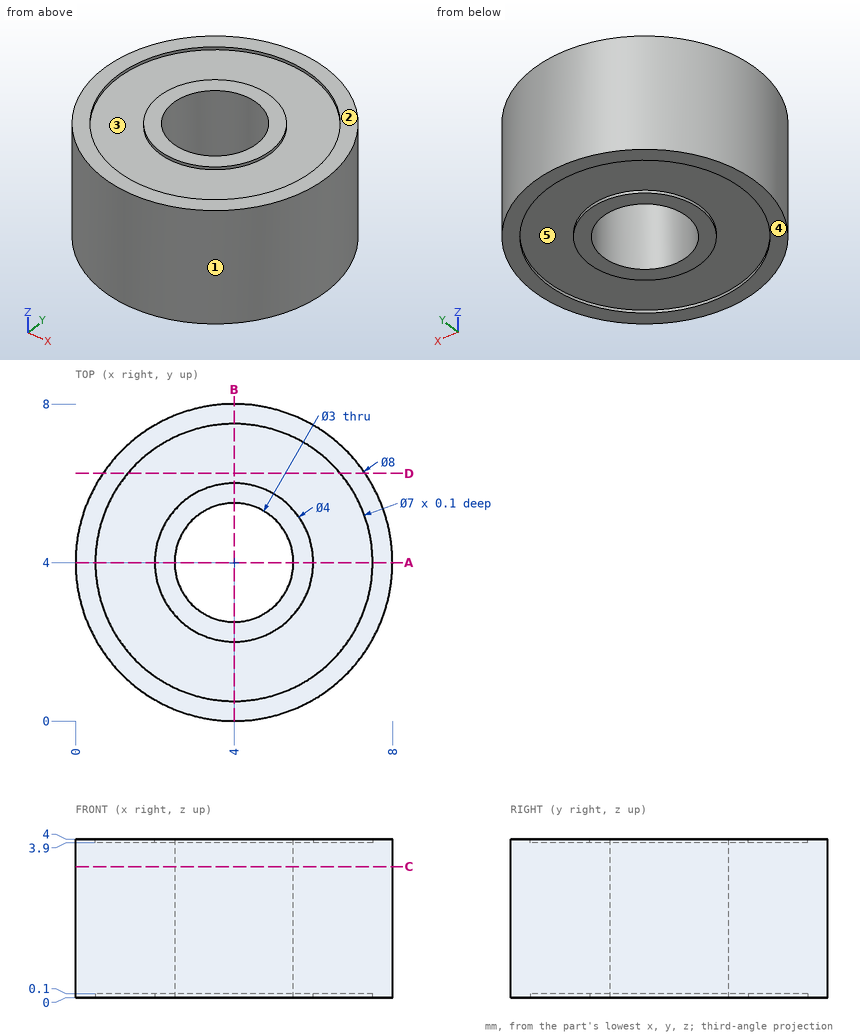
Verification items for this drawing (mm, ordinates from the low corner). A direction names the side the tool comes from. Coordinates: 2 decimals unless noted, no trailing zeros. Order: outer loops, then holes, each group sorted by start corner. A loop starts at its lowest first (then second) coordinate and runs counter-clockwise, first axis right, second up. Notation, with made-up numbers: M 38.5,30.25 L 80.5,30.25 A32 ccw 80.5,61.25 Z; hole C 21.25,79 d9. An arc over 180 degrees is marked long. Answer as a JSON object with one key per item and string values.
Q1. Cross-section at D-D on y = 6.25. Record the cut outline in (x, z).
Results are:
{"outline": "M 0.69,0 L 1.32,0 L 1.32,0.1 L 6.68,0.1 L 6.68,0 L 7.31,0 L 7.31,4 L 6.68,4 L 6.68,3.9 L 1.32,3.9 L 1.32,4 L 0.69,4 Z"}
Q2. Release check for a two-part mould opening along Y. For the marked faces 1, 2 and 3 record: released by +Y, released by -Y, zero draft, split by the parting line, or undercut.
Results are:
{"face 1": "split by the parting line", "face 2": "zero draft", "face 3": "undercut"}
Q3. Cross-section at A-A on y = 4. Record the cut outline in (x, z), and give its area (3 significant figures).
Results are:
{"outline": "M 0,0 L 0.5,0 L 0.5,0.1 L 2,0.1 L 2,0 L 2.5,0 L 2.5,4 L 2,4 L 2,3.9 L 0.5,3.9 L 0.5,4 L 0,4 Z; M 5.5,0 L 6,0 L 6,0.1 L 7.5,0.1 L 7.5,0 L 8,0 L 8,4 L 7.5,4 L 7.5,3.9 L 6,3.9 L 6,4 L 5.5,4 Z", "area": "19.4 mm²"}
Q4. Cross-section at C-C on z = 3.3. Record the cut outline in (x, y).
Results are:
{"outline": "C 4,4 d8; hole C 4,4 d3"}
Q5. Tool access check on the marked faces 4 and 5. Record the directions out of +Z, -Z, +X, -X, +Y, -Y that give a thin tool (end or side, any length) a straight path to the whole face; none if there is none.
Results are:
{"face 4": "-Z, +X, -X, +Y, -Y", "face 5": "-Z"}
Q6. Scan lines: line 1 (Y direction, x = 4, z = 0.05); line 2 (Y direction, x = 4, z = 2.25); line 3 (Z direction, x = 5, y = 6.75). Record each from-to range of solid material in increasing order.
Results are:
{"line 1": "y = 0 to 0.5, 2 to 2.5, 5.5 to 6, 7.5 to 8", "line 2": "y = 0 to 2.5, 5.5 to 8", "line 3": "z = 0.1 to 3.9"}
Q7. Depth check by flat-ended pin: pin 1 Ø2 at (x, y) = (2.5, 5) entering from -Z; pin 2 Ø2 at (y, z) = (5.5, 3) entering from -X; pin 3 Ø1 at (y, z) = (2, 1.5) entering from +X. Enter the tip coordinate at first touch or a pass-through.
Results are:
{"pin 1": "stops at z = 0", "pin 2": "stops at x = 0.03", "pin 3": "stops at x = 7.71"}
